from build123d import *

# Parameters (mm, degrees)
SKETCH_1_W          = 80
SKETCH_1_H          = 150
SKETCH_1_R          = 1.5
EXTRUDE_1_DEPTH     = 3
CUT_EXTRUDE_START   = -10
CUT_EXTRUDE_1_DEPTH = 10
SKETCH_3_R          = 2
CUT_EXTRUDE_2_DEPTH = 10
SKETCH_4_W          = 87.19
SKETCH_4_H          = 8
CUT_EXTRUDE_3_DEPTH = 10
FILLET_1_R          = 10


with BuildPart() as part:
    # 草图1 → 凸台-拉伸1 (new body)
    with BuildSketch(Plane.XY):
        Rectangle(SKETCH_1_W, SKETCH_1_H)
        with Locations((24, 0)):
            Circle(SKETCH_1_R, mode=Mode.SUBTRACT)
        with Locations(Location((-24, 0, 0), (0, 0, 180))):
            Circle(SKETCH_1_R, mode=Mode.SUBTRACT)
        with Locations((24.5, 48)):
            Circle(SKETCH_1_R, mode=Mode.SUBTRACT)
        with Locations((-24.5, 48)):
            Circle(SKETCH_1_R, mode=Mode.SUBTRACT)
        with Locations((26, -58)):
            Circle(SKETCH_1_R, mode=Mode.SUBTRACT)
        with Locations((-26, -58)):
            Circle(SKETCH_1_R, mode=Mode.SUBTRACT)
    extrude(amount=EXTRUDE_1_DEPTH)

    # 草图2 → 切除-拉伸1 (cut)
    with BuildSketch(Plane.XY.offset(3).offset(CUT_EXTRUDE_START)):
        with BuildLine():
            Line((-27.5, -58), (-27.5, -46))
            ThreePointArc((-27.5, -46), (-26, -44.5), (-24.5, -46))
            Line((-24.5, -46), (-24.5, -58))
            ThreePointArc((-24.5, -58), (-26, -59.5), (-27.5, -58))
        make_face()
        with BuildLine():
            Line((27.5, -58), (27.5, -46))
            ThreePointArc((27.5, -46), (26, -44.5), (24.5, -46))
            Line((24.5, -46), (24.5, -58))
            ThreePointArc((24.5, -58), (26, -59.5), (27.5, -58))
        make_face()
    extrude(amount=CUT_EXTRUDE_1_DEPTH, mode=Mode.SUBTRACT)

    # 草图3 → 切除-拉伸2 (cut)
    with BuildSketch(Plane.XY.offset(3)):
        with Locations((24.5, 58)):
            Circle(SKETCH_3_R)
        with Locations((24.5, 48)):
            Circle(SKETCH_3_R)
        with Locations((-24.5, 48)):
            Circle(SKETCH_3_R)
        with Locations((-24.5, 58)):
            Circle(SKETCH_3_R)
    extrude(amount=-CUT_EXTRUDE_2_DEPTH, mode=Mode.SUBTRACT)

    # 草图4 → 切除-拉伸3 (cut)
    with BuildSketch(Plane.XY.offset(3)):
        with Locations((3.595, 71)):
            Rectangle(SKETCH_4_W, SKETCH_4_H)
    extrude(amount=-CUT_EXTRUDE_3_DEPTH, mode=Mode.SUBTRACT)

    # 圆角1
    fillet_1_edges = [part.edges().sort_by_distance(p)[0] for p in [
        (-40, 67, 1.5),
        (40, 67, 1.5),
        (40, -75, 1.5),
        (-40, -75, 1.5),
    ]]
    fillet(fillet_1_edges, radius=FILLET_1_R)


solid = part.part
Build history of the part. All positions in model axes, mm. A direction names the side the tool comes from. Round coordinates to 2 decimals unless told otherwise and drop trailing zeros. Loops run counter-clockwise (first coordinate to the right, second up) from the corner with the lowest first, then second, coordinate; pieces in that order, holes last. Notation, with made-up numbers: (14, -11) -> (46, -11) arc R28 cw to (46, 10) -> close; hole circle Ø11 at (-10.75, -14.5). An arc over 180 degrees is marked (long way). One line per item, written item: value. Start each with the question number.
Q1. Two-plate mould, pull along X, no slides. Class faces 1 (the face through (24.5, -52, 1)), 2 (the face through (0, 67, 2)), 3 (the face through (40, -5, 1)): released by +X, released by -X, zero draft, split by the parting line, or undercut.
Q2. Cut at B-B on z = 1. Count the separate pieces of the cut face and the enclosed holes in it, plus the area to 3 significant figures.
Q3. 3-axis set-ups, long thin cutter, end or side, ignore diameter. For faces 4 (the face through (-26, -59.5, 1.5)), 5 (the face through (-1, -3, 3)): which of +Z, -Z, +X, -X, +Y, -Y reach the whole face in a straight line?
Q4. Cut at A-A on y = 0. List the corners of the cut face in (x, z), plus the area to 3 significant figures.
Q5. Probe line 1 along X through (y, z) = (-54.5, 1.85); line 2 along Y through (x, z) = (-24, 1.9); line 3 along Y through (x, z) = (-23, 1.7). List the from-to ranges inside material, lowest first.
Computed:
1. face 1: undercut
1. face 2: zero draft
1. face 3: released by +X
2. separate pieces: 1
2. enclosed holes: 8
2. area: 11,100 mm²
3. face 4: +Z, -Z
3. face 5: +Z, +X, -X, +Y, -Y
4. outline: (-40, 0) -> (-25.5, 0) -> (-25.5, 3) -> (-40, 3) -> close; (-22.5, 0) -> (22.5, 0) -> (22.5, 3) -> (-22.5, 3) -> close; (25.5, 0) -> (40, 0) -> (40, 3) -> (25.5, 3) -> close
4. area: 222 mm²
5. line 1: -40 to -27.5, -24.5 to 24.5, 27.5 to 40
5. line 2: -75 to -1.5, 1.5 to 46.06, 49.94 to 56.06, 59.94 to 67
5. line 3: -75 to -1.12, 1.12 to 46.68, 49.32 to 56.68, 59.32 to 67
